from build123d import *

# Parameters (mm, degrees)
SKETCH_R     = 40
PAD_DEPTH    = 100
SKETCH001_R  = 39.5
PAD001_DEPTH = 12
SKETCH002_R  = 35.75
PAD002_DEPTH = 12
SKETCH003_R  = 17
PAD003_DEPTH = 56
SKETCH004_R  = 3
PAD004_DEPTH = 22


with BuildPart() as part:
    # Sketch → Pad (new body)
    with BuildSketch(Plane.XY):
        Circle(SKETCH_R)
    extrude(amount=-PAD_DEPTH)

    # Sketch001 (on Face3 of Pad) → Pad001 (join)
    with BuildSketch(Plane(origin=(0, 0, -100), x_dir=(1, 0, 0), z_dir=(0, 0, -1))):
        Circle(SKETCH001_R)
    extrude(amount=PAD001_DEPTH)

    # Sketch002 (on Face5 of Pad001) → Pad002 (join)
    with BuildSketch(Plane(origin=(0, 0, -112), x_dir=(1, 0, 0), z_dir=(0, 0, -1))):
        Circle(SKETCH002_R)
    extrude(amount=PAD002_DEPTH)

    # Sketch003 (on Face7 of Pad002) → Pad003 (join)
    with BuildSketch(Plane(origin=(0, 0, -124), x_dir=(1, 0, 0), z_dir=(0, 0, -1))):
        Circle(SKETCH003_R)
    extrude(amount=PAD003_DEPTH)

    # Sketch004 (on Face9 of Pad003) → Pad004 (join)
    with BuildSketch(Plane(origin=(0, 0, -180), x_dir=(1, 0, 0), z_dir=(0, 0, -1))):
        Circle(SKETCH004_R)
    extrude(amount=PAD004_DEPTH)


solid = part.part
Here's how the part is built. I have some questions about the finished solid (model axes, mm). A direction names the side the tool comes from. Give positions to 0.01 mm unless a question says otherwise; leave off trailing zeros. Loops run counter-clockwise (first coordinate to the right, second up) from the corner with the lowest first, then second, coordinate; pieces in that order, holes last. Notation, with made-up numbers: (85, 24) -> (92, 24) arc R13 cw to (92, 32) -> close; hole circle Ø6 at (35, 58.25). An arc over 180 degrees is marked (long way). Answer as a JSON object with one key per item and string values. Group by question number.
Item 1: On a 3-axis mill with a long thin cutter (end or side, diameter ignored), from which of +Z, -Z, +X, -X, +Y, -Y can I reach the whole of each face in a straight line? I mean faces 1 (the cylindrical face through (-29.11, -26.7, -105.92)), 2 (the flat face through (-1, 1, 0)). Say none if no direction works.
Item 2: Imagine slicing it at C-C on z = -77. Write out the boundary of the cut face in (x, y), then the cut area to 3 significant figures.
Item 3: I need wall thicknesses on L1, parallel to X at y = 0, z = -153; L2, parallel to Z at x = 30, y = 17; L3, parallel to Y at x = -0.5, z = -175. Which ranges of each line are inside material? Lowest first, please.
Item 4: Will these pins go through, and if not, where does the flat tip stop? pin 1 (1.5 mm diameter, centred on x = -12, y = -31.5, fed in from +Z); pin 2 (5 mm diameter, centred on y = 6, z = -62, fed in from +X); pin 3 (6 mm diameter, centred on y = 29.5, z = -40.5, fed in from +X); pin 4 (10 mm diameter, centred on y = -29.5, z = -92.5, fed in from -X).
Item 5: Imagine slicing it at B-B on y = -24.5. Write out the boundary of the cut face in (x, z), then the cut area to 3 significant figures.
Item 6: Imagine slicing it at A-A on x = 0. Write out the boundary of the cut face in (y, z).
Answer list:
{
 "1": {"face 1": "-Z", "face 2": "+Z, +X, -X, +Y, -Y"},
 "2": {"outline": "circle Ø80 at (0, 0)", "area": "5,030 mm2"},
 "3": {"L1": "x = -17 to 17", "L2": "z = -124 to 0", "L3": "y = -16.99 to 16.99"},
 "4": {"pin 1": "stops at z = 0", "pin 2": "stops at x = 39.85", "pin 3": "stops at x = 29.96", "pin 4": "stops at x = -31.62"},
 "5": {"outline": "(-31.62, -100) -> (-30.98, -100) -> (-30.98, -112) -> (-26.03, -112) -> (-26.03, -124) -> (26.03, -124) -> (26.03, -112) -> (30.98, -112) -> (30.98, -100) -> (31.62, -100) -> (31.62, 0) -> (-31.62, 0) -> close", "area": "7,690 mm2"},
 "6": {"outline": "(-40, -100) -> (-39.5, -100) -> (-39.5, -112) -> (-35.75, -112) -> (-35.75, -124) -> (-17, -124) -> (-17, -180) -> (-3, -180) -> (-3, -202) -> (3, -202) -> (3, -180) -> (17, -180) -> (17, -124) -> (35.75, -124) -> (35.75, -112) -> (39.5, -112) -> (39.5, -100) -> (40, -100) -> (40, 0) -> (-40, 0) -> close"}
}
